Build history of the part. All positions in model axes, mm. A direction names the side the tool comes from. Round coordinates to 2 decimals unless told otherwise and drop trailing zeros. Write each loop counter-clockwise with the first axis right and the second up, starting at its lowest first coordinate (ties: lowest second). Pieces come first, ordered by that corner, then holes.
1) Flat gauge pins, fed straight in: pin 1 (5 mm diameter, centred on x = 22, z = 3, fed in from +Y); pin 2 (5.5 mm diameter, centred on x = 42.5, y = -42.5, fed in from +Z); pin 3 (1.5 mm diameter, centred on y = 20.5, z = 1.5, fed in from +X). Where does each tip first touch, or does it go through?
2) Pull direction Y, two halves, no side cores. Call faces 3 (the flat face through (0, 0, 0)), 4 (the flat face through (-1, 1, -3.5)), 5 (the cylindrical face through (17.535, 33.713, 2.958)), 6 (the cylindrical face through (41.284, -41.385, -1.726)): +Y half, -Y half, draft (parallel to the pull), parting line (faces both ways), or undercut.
3) Saw through at C-C (x = 0). Write the cut outline in (y, z), plus the area to 3 significant figures.
4) Which spindle directions (+Z, -Z, +X, -X, +Y, -Y) get a long thin tool onto all of the face, cutting with end or side? Do faces 1 (the cylindrical face through (-29.97, -1.32, 4.12)), 2 (the flat face through (50, -1, -2)). Say none if no direction does.
5) Saw through at A-A (x = -42.5). Write the cut outline in (y, z), plus the area to 3 significant figures.
6) Wall check: probe 1 along Y at (x, z) = (42.5, -1.35); probe 2 along Z at (x, y) = (-4, 44); probe 3 along X at (y, z) = (-11, 2.25). Give the ranges that are in metal, low to high.
Solid Edge part; units mm, degrees
sketch "Sketch1" plane through (0, 0, 0) normal (0, 0, 1) x (1, 0, 0)
  circle A0 centre (42.5, 42.5) radius 1.65
  circle A1 centre (-42.5, 42.5) radius 1.65
  circle A2 centre (-42.5, -42.5) radius 1.65
  circle A3 centre (42.5, -42.5) radius 1.65
  line L0 (50, 50) -> (-50, 50)
  line L1 (-50, 50) -> (-50, -50)
  line L2 (-50, -50) -> (50, -50)
  line L3 (50, -50) -> (50, 50)
extrude "Protrusion1" add sketch "Sketch1" against normal blind 3.5
sketch "Sketch2" plane through (0, 0, 0) normal (0, 0, 1) x (1, 0, 0)
  circle A0 centre (0, 0) radius 30
  circle A1 centre (0, 0) radius 38
extrude "ExtrudedProtrusion_2" add sketch "Sketch2" along normal blind 6.5
chamfer "Chamfer_1" distance 0.5 angle 45 1 edges at (-38, 0, 6.5)
chamfer "Chamfer_2" distance 1.8 angle 45 1 edges at (-30, 0, 0)
Evaluation:
1. pin 1: stops at y = 32.62
1. pin 2: stops at z = 0
1. pin 3: stops at x = 32.46
2. face 3: undercut
2. face 4: draft
2. face 5: parting line
2. face 6: undercut
3. outline: (-50, -3.5) - (50, -3.5) - (50, 0) - (38, 0) - (38, 6) - (37.5, 6.5) - (30, 6.5) - (30, 1.8) - (28.2, 0) - (-28.2, 0) - (-30, 1.8) - (-30, 6.5) - (-37.5, 6.5) - (-38, 6) - (-38, 0) - (-50, 0) - close
3. area: 457 mm2
4. face 1: +Z
4. face 2: +Z, -Z, +X, +Y, -Y
5. outline: (-50, -3.5) - (-44.15, -3.5) - (-44.15, 0) - (-50, 0) - close; (-40.85, -3.5) - (40.85, -3.5) - (40.85, 0) - (-40.85, 0) - close; (44.15, -3.5) - (50, -3.5) - (50, 0) - (44.15, 0) - close
5. area: 327 mm2
6. probe 1: y = -50 to -44.15, -40.85 to 40.85, 44.15 to 50
6. probe 2: z = -3.5 to 0
6. probe 3: x = -36.37 to -27.91, 27.91 to 36.37
